Could you check a few things on this model? Use its own coordinates, in mm. Give positions to 0.01 mm unless a question says otherwise; leave off trailing zeros. Write each loop counter-clockwise with the first axis right and the second up, starting at its lowest first coordinate (ties: lowest second). Pieces come first, ordered by that corner, then holes. Notation, with made-up numbers: M 50,-16 L 62,-16 A32 ccw 62,21 Z; hole C 53,88 d8. An arc over 180 degrees is marked long. Use one line per item in the form item = value.
from build123d import *

# Parameters (mm, degrees)
BOSS_EXTRUDE2_DEPTH      = 3.048
SKETCH2_R                = 1.143
CUT_EXTRUDE1_DEPTH       = 101.398460187
SKETCH4_R                = 38.1
CUT_EXTRUDE3_DEPTH       = 124.46
FILLET1_R                = 6.35
SKETCH12_R               = 1.651
CUT_EXTRUDE11_DEPTH      = 75.692
SKETCH14_R               = 1.651
CUT_EXTRUDE13_DEPTH      = 97.79
SKETCH15_R               = 3.175
CUT_EXTRUDE14_DEPTH      = 103.378
CUT_EXTRUDE14_DEPTH_BACK = 48.768
SKETCH3_R                = 12.1285
SKETCH3_R_2              = 12.192
CUT_EXTRUDE2_DEPTH       = 101.398460332
FILLET2_R                = 2.54


with BuildPart() as part:
    # Sketch1 → Boss-Extrude2 (new body)
    with BuildSketch(Plane.XY):
        with BuildLine():
            Line((-66.753693561, 34.036), (-54.815693561, 34.036))
            Line((-54.815693561, 34.036), (-54.815693561, -34.036))
            Line((-54.815693561, -34.036), (-66.753693561, -34.036))
            ThreePointArc((-66.753693561, -34.036), (0, -74.93), (66.753693561, -34.036))
            Line((66.753693561, -34.036), (54.815693561, -34.036))
            Line((54.815693561, -34.036), (54.815693561, 34.036))
            Line((54.815693561, 34.036), (66.753693561, 34.036))
            ThreePointArc((66.753693561, 34.036), (0, 74.93), (-66.753693561, 34.036))
        make_face()
    extrude(amount=BOSS_EXTRUDE2_DEPTH)

    # Sketch2 → Cut-Extrude1 (cut, through all)
    with BuildSketch(Plane.XY.offset(3.048)):
        with Locations((-6.731, 62.23)):
            Circle(SKETCH2_R)
        with Locations((6.731, 62.23)):
            Circle(SKETCH2_R)
    extrude(amount=-CUT_EXTRUDE1_DEPTH, mode=Mode.SUBTRACT)

    # Sketch4 → Cut-Extrude3 (cut)
    with BuildSketch(Plane(origin=(0, 0, 0), x_dir=(-1, 0, 0), z_dir=(0, 0, -1))):
        with Locations((0, -86.312058398)):
            Circle(SKETCH4_R)
    extrude(amount=-CUT_EXTRUDE3_DEPTH, mode=Mode.SUBTRACT)

    # Fillet1
    fillet1_edges = [part.edges().sort_by_distance(p)[0] for p in [
        (-33.000960548, -67.271401821, 1.524),
        (33.000960548, -67.271401821, 1.524),
    ]]
    fillet(fillet1_edges, radius=FILLET1_R)

    # Sketch12 → Cut-Extrude11 (cut)
    with BuildSketch(Plane(origin=(30.092005081, 4.08352975, 0), x_dir=(-1, 0, 0), z_dir=(0, 0, -1))):
        with Locations((63.757223581, 17.50647025)):
            Circle(SKETCH12_R)
        with Locations((63.757223581, -25.67352975)):
            Circle(SKETCH12_R)
        with Locations((-3.552776419, -25.67352975)):
            Circle(SKETCH12_R)
        with Locations((-3.552776419, 17.50647025)):
            Circle(SKETCH12_R)
    extrude(amount=-CUT_EXTRUDE11_DEPTH, mode=Mode.SUBTRACT)

    # Sketch14 → Cut-Extrude13 (cut)
    with BuildSketch(Plane(origin=(30.092005081, 4.08352975, -30.0355), x_dir=(-1, 0, 0), z_dir=(0, 0, -1))):
        with Locations(Location((4.154396091, -49.728759131, 0), (0, 0, 180))):
            Circle(SKETCH14_R)
        with Locations(Location((56.02961407, -49.728759131, 0), (0, 0, 180))):
            Circle(SKETCH14_R)
        with Locations(Location((4.154396091, 41.38247025, 0), (0, 0, 180))):
            Circle(SKETCH14_R)
        with Locations(Location((56.02961407, 41.38247025, 0), (0, 0, 180))):
            Circle(SKETCH14_R)
    extrude(amount=-CUT_EXTRUDE13_DEPTH, mode=Mode.SUBTRACT)

    # Sketch15 → Cut-Extrude14 (cut, two sides)
    with BuildSketch(Plane(origin=(30.092005081, 4.08352975, 6.096), x_dir=(-1, 0, 0), z_dir=(0, 0, -1))) as cut_extrude14_sk:
        with Locations(Location((-16.897994919, 21.31647025, 0), (0, 0, 180))):
            Circle(SKETCH15_R)
        with Locations(Location((77.082005081, 21.31647025, 0), (0, 0, 180))):
            Circle(SKETCH15_R)
        with Locations(Location((30.092005081, 21.31647025, 0), (0, 0, 180))):
            Circle(SKETCH15_R)
        with Locations(Location((77.082005081, -29.48352975, 0), (0, 0, 180))):
            Circle(SKETCH15_R)
        with Locations(Location((30.092005081, -29.48352975, 0), (0, 0, 180))):
            Circle(SKETCH15_R)
        with Locations(Location((-16.897994919, -29.48352975, 0), (0, 0, 180))):
            Circle(SKETCH15_R)
    extrude(amount=CUT_EXTRUDE14_DEPTH, mode=Mode.SUBTRACT)
    extrude(cut_extrude14_sk.sketch, amount=-CUT_EXTRUDE14_DEPTH_BACK, mode=Mode.SUBTRACT)

    # Sketch3 → Cut-Extrude2 (cut, through all)
    with BuildSketch(Plane(origin=(0, 0, 0), x_dir=(-1, 0, 0), z_dir=(0, 0, -1))):
        with Locations((-31.75, 0)):
            Circle(SKETCH3_R)
        with Locations((31.75, 0)):
            Circle(SKETCH3_R)
        Circle(SKETCH3_R_2)
        with Locations((-43.105229381, -43.105229381)):
            Circle(SKETCH3_R)
        with Locations((14.224, -34.29)):
            Circle(SKETCH3_R)
        with Locations((14.224, 34.29)):
            Circle(SKETCH3_R)
        with Locations((-43.105229381, 43.105229381)):
            Circle(SKETCH3_R)
        with Locations((43.105229381, 43.105229381)):
            Circle(SKETCH3_R)
        with Locations((-14.224, 34.29)):
            Circle(SKETCH3_R)
        with Locations((-14.224, -34.29)):
            Circle(SKETCH3_R)
        with Locations((43.105229381, -43.105229381)):
            Circle(SKETCH3_R)
        with BuildLine():
            Line((7.62, 15.24), (-7.62, 15.24))
            ThreePointArc((-7.62, 15.24), (-16.292102448, 11.647897552), (-12.7, 20.32))
            Line((-12.7, 20.32), (-8.107123288, 22.407671233))
            ThreePointArc((-8.107123288, 22.407671233), (-4.600183073, 23.292845139), (-2.54, 20.32))
            Line((-2.54, 20.32), (2.54, 20.32))
            ThreePointArc((2.54, 20.32), (4.600183073, 23.292845139), (8.107123288, 22.407671233))
            Line((8.107123288, 22.407671233), (12.7, 20.32))
            ThreePointArc((12.7, 20.32), (16.292102448, 11.647897552), (7.62, 15.24))
        make_face()
        with BuildLine():
            Line((7.62, -15.24), (-7.62, -15.24))
            ThreePointArc((-7.62, -15.24), (-16.292102448, -11.647897552), (-12.7, -20.32))
            Line((-12.7, -20.32), (-8.107123288, -22.407671233))
            ThreePointArc((-8.107123288, -22.407671233), (-4.600183073, -23.292845139), (-2.54, -20.32))
            Line((-2.54, -20.32), (2.54, -20.32))
            ThreePointArc((2.54, -20.32), (4.600183073, -23.292845139), (8.107123288, -22.407671233))
            Line((8.107123288, -22.407671233), (12.7, -20.32))
            ThreePointArc((12.7, -20.32), (16.292102448, -11.647897552), (7.62, -15.24))
        make_face()
    extrude(amount=-CUT_EXTRUDE2_DEPTH, mode=Mode.SUBTRACT)

    # Fillet2
    fillet2_edges = [part.edges().sort_by_distance(p)[0] for p in [
        (-7.62, -15.24, 1.524),
        (-2.54, -20.32, 1.524),
        (2.54, -20.32, 1.524),
        (7.62, -15.24, 1.524),
        (-7.62, 15.24, 1.524),
        (7.62, 15.24, 1.524),
        (2.54, 20.32, 1.524),
        (-2.54, 20.32, 1.524),
    ]]
    fillet(fillet2_edges, radius=FILLET2_R)


solid = part.part
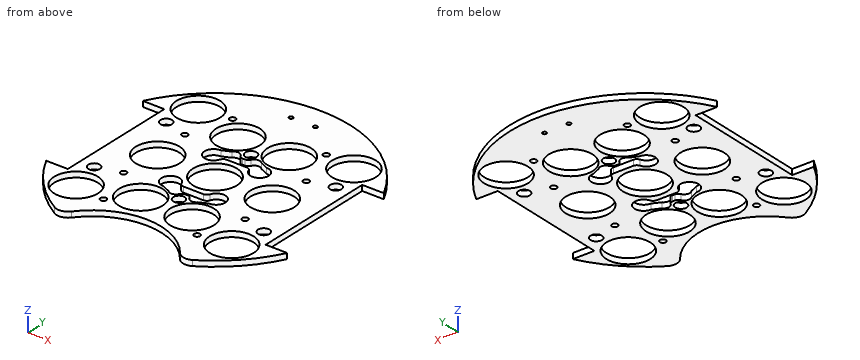
1) I want a section at C-C, the plane z = 2.1. Count the separate pieces of the cut face and the enclosed holes in it, plus the area to 3 significant figures.
Checked values:
separate_pieces = 1
enclosed_holes = 29
area = 8,080 mm2
2) I want a section at A-A, the plane y = -25.4. Please give me the cut outline in (x, z) (3 decimals).
Checked values:
outline = M -54.816,0 L -50.165,0 L -50.165,3.048 L -54.816,3.048 Z; M -43.815,0 L -22.474,0 L -22.474,3.048 L -43.815,3.048 Z; M -5.974,0 L -3.175,0 L -3.175,3.048 L -5.974,3.048 Z; M 3.175,0 L 5.974,0 L 5.974,3.048 L 3.175,3.048 Z; M 22.474,0 L 43.815,0 L 43.815,3.048 L 22.474,3.048 Z; M 50.165,0 L 54.816,0 L 54.816,3.048 L 50.165,3.048 Z
3) If I drill on L1, parallel to Y at x = 0, z = 2 (3 decimals); L2, parallel to Y at x = -39.5, z = 0.7; L3, parallel to Y at x = -48, z = 2.45, over which ranges is the centre line in solid material (lowest first)?
Checked values:
L1 = -48.212 to -28.575, -22.225 to -20.32, -15.24 to -12.192, 12.192 to 15.24, 20.32 to 22.225, 28.575 to 74.93
L2 = -63.67 to -54.69, -31.52 to -9.33, 9.33 to 31.52, 54.69 to 63.67
L3 = -57.54 to -54.2, -32.01 to -28.41, -22.39 to 22.39, 28.41 to 32.01, 54.2 to 57.54
4) For pin 1 Ø1.5 at (x, z) = (-2.5, 2) entering from +Y; pin 2 Ø1.5 at (y, z) = (42.5, 2.5) entering from +X; pin 3 Ø0.9 at (y, z) = (11, 1.5) entering from -X, each with a flat end and sliding along its axis, tell me the tip position at first contact or that it passes through.
Checked values:
pin_1 = 74.91
pin_2 = 62.22
pin_3 = -54.82
5) I want a section at B-B, the plane x = 21.5. Please give me the cut outline in (y, z).
Checked values:
outline = M -54.86,0 L -43.99,0 L -43.99,3.05 L -54.86,3.05 Z; M -24.59,0 L -6.48,0 L -6.48,3.05 L -24.59,3.05 Z; M 6.48,0 L 24.59,0 L 24.59,3.05 L 6.48,3.05 Z; M 43.99,0 L 71.78,0 L 71.78,3.05 L 43.99,3.05 Z
